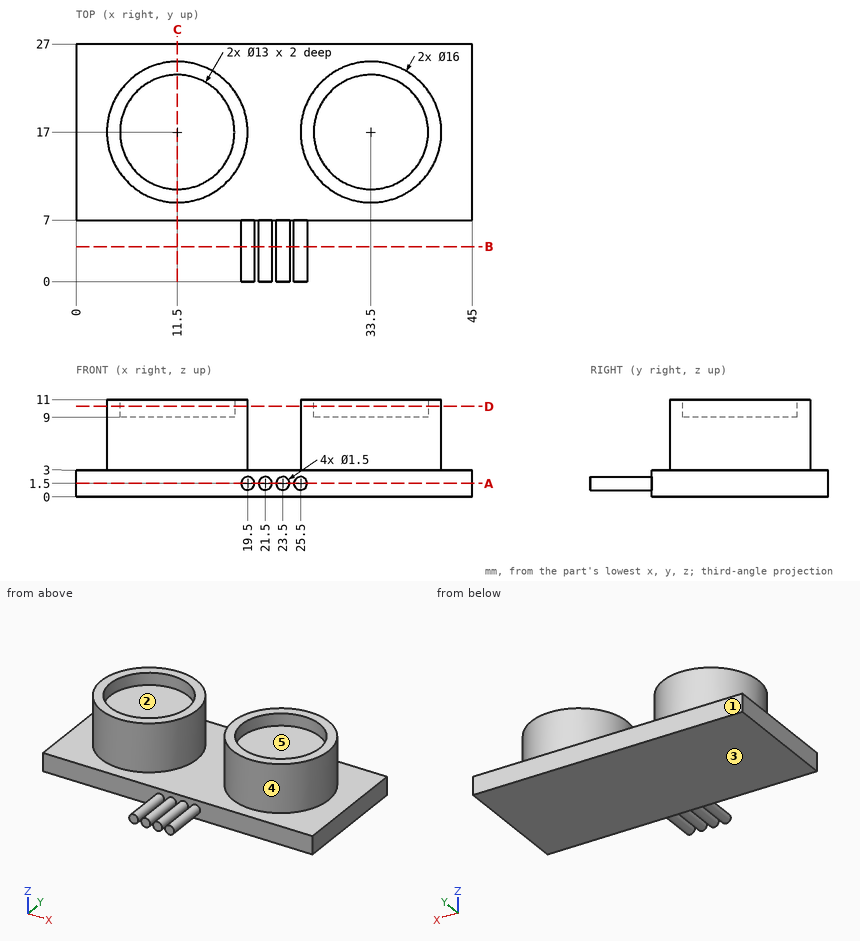
Design review of the part shown in the three views and the two pictorial views. Dimensions are in mm from the part's minimum x, y and z. A direction names the side the tool comes from. Round coordinates to 2 decimals unless told otherwise and drop trailing zeros. Write each loop counter-clockwise with the first axis right and the second up, starting at its lowest first coordinate (ties: lowest second). Pieces come first, ordered by that corner, then holes. Notation, with made-up numbers: (8.25, 7) -> (18.25, 7) arc R24 ccw to (18.25, 38) -> close; hole circle Ø9 at (38, 72). An arc over 180 degrees is marked (long way). Use one line per item in the form item = value.
1) Take a section at D-D, the plane z = 10.25. Write out the cut boundary in (x, y).
Found:
outline = circle Ø16 at (11.5, 17); circle Ø16 at (33.5, 17); hole circle Ø13 at (11.5, 17); hole circle Ø13 at (33.5, 17)
2) Clearance check with flat-ended pins moving along their axes: pin 1 (5 mm diameter, centred on x = 13, z = 7.5, fed in from +Y); pin 2 (8 mm diameter, centred on x = 33.5, y = 17, fed in from +Z); pin 3 (2 mm diameter, centred on x = 21, y = 4, fed in from +Z). State where each tip first meets the part, or that it passes through.
Found:
pin_1 = 25
pin_2 = 9
pin_3 = 2.25
3) Take a section at B-B, the plane y = 4. Write out the cut boundary in (x, z).
Found:
outline = circle Ø1.5 at (19.5, 1.5); circle Ø1.5 at (21.5, 1.5); circle Ø1.5 at (23.5, 1.5); circle Ø1.5 at (25.5, 1.5)
4) Tool access review of the marked faces 1 and 2: name each direction out of +Z, -Z, +X, -X, +Y, -Y from which nothing blocks a thin tool from reaching the whole face with its end or side.
Found:
face_1 = +Z, -Z, +X, -X, +Y
face_2 = +Z
5) Take a section at C-C, the plane x = 11.5. Write out the cut boundary in (y, z), and give its area (3 significant figures).
Found:
outline = (7, 0) -> (27, 0) -> (27, 3) -> (25, 3) -> (25, 11) -> (23.5, 11) -> (23.5, 9) -> (10.5, 9) -> (10.5, 11) -> (9, 11) -> (9, 3) -> (7, 3) -> close
area = 162 mm2
6) Mouldability with a two-part tool opening along Y and no side actions: class the marked faces 3, 4 and 5 as +Y half, -Y half, draft (parallel to the pull), parting line (faces both ways), or undercut.
Found:
face_3 = draft
face_4 = parting line
face_5 = undercut
7) To check wall thickness, follow L1, parallel to Y at x = 11.5, z = 10.3; L2, parallel to X at y = 22.75, z = 10; L3, parallel to X at y = 3.5, z = 2. State the ranges of each line that lie inside material, in increasing order. Write a range as from..to.
Found:
L1 = 9..10.5, 23.5..25
L2 = 5.94..8.47, 14.53..17.06, 27.94..30.47, 36.53..39.06
L3 = 18.94..20.06, 20.94..22.06, 22.94..24.06, 24.94..26.06
8) Take a section at A-A, the plane z = 1.5. Write out the cut boundary in (x, y).
Found:
outline = (0, 7) -> (18.75, 7) -> (18.75, 0) -> (20.25, 0) -> (20.25, 7) -> (20.75, 7) -> (20.75, 0) -> (22.25, 0) -> (22.25, 7) -> (22.75, 7) -> (22.75, 0) -> (24.25, 0) -> (24.25, 7) -> (24.75, 7) -> (24.75, 0) -> (26.25, 0) -> (26.25, 7) -> (45, 7) -> (45, 27) -> (0, 27) -> close
